Build history of the part. All positions in model axes, mm. A direction names the side the tool comes from. Round coordinates to 2 decimals unless told otherwise and drop trailing zeros. Loops run counter-clockwise (first coordinate to the right, second up) from the corner with the lowest first, then second, coordinate; pieces in that order, holes last. Notation, with made-up numbers: M -29,31.5 L 8,31.5 A35 ccw 8,69.5 Z; hole C 4,-38.75 d8. An arc over 180 degrees is marked long. Write each question's results on one line, items separated by ' | '. Start each with the question number.
Autodesk Inventor part; units mm, degrees
ref_plane "YZ Plane" through (0, 0, 0) normal (1, 0, 0) x (0, 1, 0)
ref_plane "XZ Plane" through (0, 0, 0) normal (0, 1, 0) x (-1, 0, 0)
ref_plane "XY Plane" through (0, 0, 0) normal (0, 0, 1) x (1, 0, 0)
sketch "スケッチ2" plane through (0, 0, 0) normal (0, 0, 1) x (1, 0, 0)
  line L0 (-46.15, -15.85) -> (46.15, -15.85)
  line L1 (46.15, -15.85) -> (46.15, 15.85)
  line L2 (46.15, 15.85) -> (-46.15, 15.85)
  line L3 (-46.15, 15.85) -> (-46.15, -15.85)
  line L4 (-46.15, -15.85) -> (46.15, 15.85) construction
  line L5 (46.15, -15.85) -> (-46.15, 15.85) construction
  point P0 (0, 0)
  dimension "d4" = 92.3
  dimension "d5" = 31.7
extrude "押し出し2" add sketch "スケッチ2" along normal mid plane 36.5
fillet "フィレット1" radius 2 4 edges at (46.15, 15.85, 0) (46.15, -15.85, 0) (-46.15, 15.85, 0) (-46.15, -15.85, 0)
sketch "スケッチ3" plane through (-44.15, -15.85, -18.25) normal (0, -1, 0) x (1, 0, 0)
  line L0 (-2, 36.5) -> (-2, 0)
  line L1 (0, 36.5) -> (88.3, 36.5)
  point P0 (44.15, 18.25)
  point P1 (44.15, 21)
  dimension "d9" = 46.15
  dimension "d10" = 15.5
hole "穴1" at (0, -15.85, 2.75) direction (0, 1, 0) diameter 4.9784 depth 19.05 tip angle 118
sketch "スケッチ4" plane through (0, 0, 18.25) normal (0, 0, 1) x (1, 0, 0)
  circle A0 centre (0, 0) radius 7.5
  dimension "d18" = 15
extrude "押し出し3" add sketch "スケッチ4" along normal blind 1
properties part number "zed_x_mini"
Item 1: Tool access for faces 1 (the cylindrical face through (0.95, -6.19, 0.45)), 2 (the cylindrical face through (-7.493, -0.33, 18.743)), 3 (the cylindrical face through (45.55, 15.28, -0.26)): list every direction of +Z, -Z, +X, -X, +Y, -Y with a clear straight run to the whole face (end or side of a thin tool).
Item 2: Saw through at D-D, the plane y = -10. Give the cut face in (x, z).
Item 3: Mould opens along Z. For faces 4 (the flat face through (10, 0, 18.25)), 5 (the conical face through (-0.422, 4.436, 2.844)), 6 (the flat face through (-46.15, 0, 0)) say: released by +Z, released by -Z, zero draft, split by the parting line, or undercut.
Item 4: Saw through at B-B, the plane x = -6.5. Give the cut face in (y, z), then the cut area to 3 significant figures.
Item 5: Saw through at A-A, the plane y = 0. Give the cut face in (x, z), then the cut area to 3 significant figures.
Item 6: Drill centre lines: line 1 along Z through (x, y) = (-27, 13); line 2 along Z through (x, y) = (0, -9.5); line 3 along Z through (x, y) = (0, -2.25). Where is each one in solid material? Low to high. Write a range as [from, to].
Item 7: Saw through at C-C, the plane y = 8.5. Give the cut face in (x, z).
Working result:
1) face 1: -Y | face 2: +Z | face 3: +Z, -Z, +X, +Y
2) outline: M -46.15,-18.25 L 46.15,-18.25 L 46.15,18.25 L -46.15,18.25 Z; hole C 0,2.75 d4.98
3) face 4: released by +Z | face 5: undercut | face 6: zero draft
4) outline: M -15.85,-18.25 L 15.85,-18.25 L 15.85,18.25 L 3.74,18.25 L 3.74,19.25 L -3.74,19.25 L -3.74,18.25 L -15.85,18.25 Z | area: 1,160 mm²
5) outline: M -46.15,-18.25 L 46.15,-18.25 L 46.15,18.25 L 7.5,18.25 L 7.5,19.25 L -7.5,19.25 L -7.5,18.25 L -46.15,18.25 Z; hole C 0,2.75 d4.98 | area: 3,360 mm²
6) line 1: z = [-18.25, 18.25] | line 2: z = [-18.25, 0.26], [5.24, 18.25] | line 3: z = [-18.25, 0.26], [5.24, 19.25]
7) outline: M -46.15,-18.25 L 46.15,-18.25 L 46.15,18.25 L -46.15,18.25 Z
